```python
from build123d import *

# Parameters (mm, degrees)
SKETCH_1_R          = 17.75
EXTRUDE_1_DEPTH     = 1.6
SKETCH_2_R          = 2
EXTRUDE_2_DEPTH     = 11.3
EXTRUDE_START       = 1.6
SKETCH_3_R          = 17.75
EXTRUDE_3_DEPTH     = 1.6
CUT_EXTRUDE_2_REACH = 30.989
SKETCH_5_R          = 3.5
SKETCH_5_R_2        = 1
SKETCH_6_R          = 6
EXTRUDE_4_DEPTH     = 10
SKETCH_7_R          = 3
EXTRUDE_5_DEPTH     = 15
CHAMFER_1_SIZE      = 0.5
CUT_EXTRUDE_START   = -12
CUT_EXTRUDE_3_DEPTH = 12
SKETCH_10_R         = 3
EXTRUDE_6_DEPTH     = 2.8
EXTRUDE_7_REACH     = 39.456
SKETCH_13_R         = 1.9
CUT_EXTRUDE_4_REACH = 48.801
CUT_EXTRUDE_5_REACH = 48.801
SKETCH_17_R         = 1.25
CHAMFER_2_SIZE      = 0.5
EXTRUDE_START_2     = 1.2
SKETCH_19_R         = 3
EXTRUDE_8_DEPTH     = 1.2
EXTRUDE_9_REACH     = 39.456
SKETCH_20_R         = 1.9
SKETCH_21_R         = 3
EXTRUDE_10_DEPTH    = 1.2
CUT_EXTRUDE_START_2 = -10
SKETCH_22_R         = 6
SKETCH_22_R_2       = 3
CUT_EXTRUDE_6_DEPTH = 10
SKETCH_24_R         = 3
CUT_EXTRUDE_8_DEPTH = 12


with BuildPart() as part:
    # ｽｹｯﾁ1 → ﾎﾞｽ - 押し出し1 (new body)
    with BuildSketch(Plane.XY):
        Circle(SKETCH_1_R)
    extrude(amount=EXTRUDE_1_DEPTH)

    # ｽｹｯﾁ2 → ﾎﾞｽ - 押し出し2 (add)
    with BuildSketch(Plane(origin=(0, 0, 0), x_dir=(-1, 0, 0), z_dir=(0, 0, -1))):
        with Locations(Location((0, -15.5, 0), (0, 0, 180))):
            Circle(SKETCH_2_R)
        with Locations(Location((-13.423393759, 7.75, 0), (0, 0, 180))):
            Circle(SKETCH_2_R)
        with Locations(Location((13.423393759, 7.75, 0), (0, 0, 180))):
            Circle(SKETCH_2_R)
    extrude(amount=EXTRUDE_2_DEPTH)

    # ｽｹｯﾁ3 → ﾎﾞｽ - 押し出し3 (add)
    with BuildSketch(Plane(origin=(0, 0, -11.3), x_dir=(-1, 0, 0), z_dir=(0, 0, -1)).offset(EXTRUDE_START)):
        with Locations(Location((0, 0, 0), (0, 0, 180))):
            Circle(SKETCH_3_R)
    extrude(amount=-EXTRUDE_3_DEPTH)

    # ｽｹｯﾁ5 → ｶｯﾄ - 押し出し2 (cut, up to next)
    with BuildSketch(Plane(origin=(0, 0, -12.9), x_dir=(-1, 0, 0), z_dir=(0, 0, -1)), mode=Mode.PRIVATE) as cut_extrude_2_sk1:
        Circle(SKETCH_5_R)
    cut_extrude_2_tool1 = extrude(cut_extrude_2_sk1.sketch, amount=-CUT_EXTRUDE_2_REACH, mode=Mode.PRIVATE) & part.part
    # ｽｹｯﾁ5 → ｶｯﾄ - 押し出し2 (cut, up to next)
    with BuildSketch(Plane(origin=(0, 0, -12.9), x_dir=(-1, 0, 0), z_dir=(0, 0, -1)), mode=Mode.PRIVATE) as cut_extrude_2_sk2:
        with Locations((-13.423393759, 7.75)):
            Circle(SKETCH_5_R_2)
    cut_extrude_2_tool2 = extrude(cut_extrude_2_sk2.sketch, amount=-CUT_EXTRUDE_2_REACH, mode=Mode.PRIVATE) & part.part
    # ｽｹｯﾁ5 → ｶｯﾄ - 押し出し2 (cut, up to next)
    with BuildSketch(Plane(origin=(0, 0, -12.9), x_dir=(-1, 0, 0), z_dir=(0, 0, -1)), mode=Mode.PRIVATE) as cut_extrude_2_sk3:
        with Locations((13.423393759, 7.75)):
            Circle(SKETCH_5_R_2)
    cut_extrude_2_tool3 = extrude(cut_extrude_2_sk3.sketch, amount=-CUT_EXTRUDE_2_REACH, mode=Mode.PRIVATE) & part.part
    # ｽｹｯﾁ5 → ｶｯﾄ - 押し出し2 (cut, up to next)
    with BuildSketch(Plane(origin=(0, 0, -12.9), x_dir=(-1, 0, 0), z_dir=(0, 0, -1)), mode=Mode.PRIVATE) as cut_extrude_2_sk4:
        with Locations((0, -15.5)):
            Circle(SKETCH_5_R_2)
    cut_extrude_2_tool4 = extrude(cut_extrude_2_sk4.sketch, amount=-CUT_EXTRUDE_2_REACH, mode=Mode.PRIVATE) & part.part
    add(cut_extrude_2_tool1.solids().sort_by_distance((0, 0, -12.9))[0], mode=Mode.SUBTRACT)
    add(cut_extrude_2_tool2.solids().sort_by_distance((13.423394, 7.75, -12.9))[0], mode=Mode.SUBTRACT)
    add(cut_extrude_2_tool3.solids().sort_by_distance((-13.423394, 7.75, -12.9))[0], mode=Mode.SUBTRACT)
    add(cut_extrude_2_tool4.solids().sort_by_distance((0, -15.5, -12.9))[0], mode=Mode.SUBTRACT)

    # ｽｹｯﾁ6 → ﾎﾞｽ - 押し出し4 (add)
    with BuildSketch(Plane.XY.offset(1.6)):
        with Locations((0, 7)):
            Circle(SKETCH_6_R)
    extrude(amount=EXTRUDE_4_DEPTH)

    # ｽｹｯﾁ7 → ﾎﾞｽ - 押し出し5 (add)
    with BuildSketch(Plane.XY.offset(11.6)):
        with Locations((0, 7)):
            Circle(SKETCH_7_R)
    extrude(amount=EXTRUDE_5_DEPTH)

    # 面取り1
    chamfer_1_edges = [part.edges().sort_by_distance(p)[0] for p in [
        (-3, 7, 26.6),
    ]]
    chamfer(chamfer_1_edges, length=CHAMFER_1_SIZE)

    # ｽｹｯﾁ8 → ｶｯﾄ - 押し出し3 (cut)
    with BuildSketch(Plane.XY.offset(26.6).offset(CUT_EXTRUDE_START)):
        with BuildLine():
            Line((1.658312395, 9.5), (-1.658312395, 9.5))
            ThreePointArc((-1.658312395, 9.5), (0, 10), (1.658312395, 9.5))
        make_face()
    extrude(amount=CUT_EXTRUDE_3_DEPTH, mode=Mode.SUBTRACT)

    # ｽｹｯﾁ10 → ﾎﾞｽ - 押し出し6 (add)
    with BuildSketch(Plane.XY.offset(1.6)):
        with Locations((0, -5.5)):
            Circle(SKETCH_10_R)
        with Locations((9.5, -2.377501001)):
            Circle(SKETCH_10_R)
        with Locations((-9.5, -2.377501001)):
            Circle(SKETCH_10_R)
    extrude_6 = extrude(amount=-EXTRUDE_6_DEPTH)

    # ﾐﾗｰ1: ﾎﾞｽ - 押し出し6 across plane
    add(extrude_6.mirror(Plane.XY.offset(-5.65)))

    # ｽｹｯﾁ13 → ﾎﾞｽ - 押し出し7 (add, up to next)
    with BuildSketch(Plane(origin=(0, 0, -1.2), x_dir=(-1, 0, 0), z_dir=(0, 0, -1)), mode=Mode.PRIVATE) as extrude_7_sk1:
        with Locations(Location((-9.5, -2.377501001, 0), (0, 0, 180))):
            Circle(SKETCH_13_R)
    extrude_7_tool1 = extrude(extrude_7_sk1.sketch, amount=EXTRUDE_7_REACH, mode=Mode.PRIVATE) - part.part
    # ｽｹｯﾁ13 → ﾎﾞｽ - 押し出し7 (add, up to next)
    with BuildSketch(Plane(origin=(0, 0, -1.2), x_dir=(-1, 0, 0), z_dir=(0, 0, -1)), mode=Mode.PRIVATE) as extrude_7_sk2:
        with Locations(Location((0, -5.5, 0), (0, 0, 180))):
            Circle(SKETCH_13_R)
    extrude_7_tool2 = extrude(extrude_7_sk2.sketch, amount=EXTRUDE_7_REACH, mode=Mode.PRIVATE) - part.part
    # ｽｹｯﾁ13 → ﾎﾞｽ - 押し出し7 (add, up to next)
    with BuildSketch(Plane(origin=(0, 0, -1.2), x_dir=(-1, 0, 0), z_dir=(0, 0, -1)), mode=Mode.PRIVATE) as extrude_7_sk3:
        with Locations(Location((9.5, -2.377501001, 0), (0, 0, 180))):
            Circle(SKETCH_13_R)
    extrude_7_tool3 = extrude(extrude_7_sk3.sketch, amount=EXTRUDE_7_REACH, mode=Mode.PRIVATE) - part.part
    add(extrude_7_tool1.solids().sort_by_distance((9.5, -2.377501, -1.2))[0])
    add(extrude_7_tool2.solids().sort_by_distance((0, -5.5, -1.2))[0])
    add(extrude_7_tool3.solids().sort_by_distance((-9.5, -2.377501, -1.2))[0])

    # ｽｹｯﾁ15 → ｶｯﾄ - 押し出し4 (cut, up to next)
    with BuildSketch(Plane(origin=(0, 0, -12.9), x_dir=(-1, 0, 0), z_dir=(0, 0, -1)), mode=Mode.PRIVATE) as cut_extrude_4_sk1:
        with BuildLine():
            Line((2.236067977, -3.5), (-2.236067977, -3.5))
            ThreePointArc((-2.236067977, -3.5), (-1.99347124, -3.258109634), (-1.724878724, -3.045454545))
            ThreePointArc((-1.724878724, -3.045454545), (0, -2.5), (1.724878724, -3.045454545))
            ThreePointArc((1.724878724, -3.045454545), (1.99347124, -3.258109634), (2.236067977, -3.5))
        make_face()
    cut_extrude_4_tool1 = extrude(cut_extrude_4_sk1.sketch, amount=-CUT_EXTRUDE_4_REACH, mode=Mode.PRIVATE) & part.part
    add(cut_extrude_4_tool1.solids().sort_by_distance((0, -3.093671, -12.9))[0], mode=Mode.SUBTRACT)

    # ｽｹｯﾁ17 → ｶｯﾄ - 押し出し5 (cut, up to next)
    with BuildSketch(Plane(origin=(0, 0, -12.9), x_dir=(-1, 0, 0), z_dir=(0, 0, -1)), mode=Mode.PRIVATE) as cut_extrude_5_sk1:
        with Locations((-6.569553896, 13.48484192)):
            Circle(SKETCH_17_R)
    cut_extrude_5_tool1 = extrude(cut_extrude_5_sk1.sketch, amount=-CUT_EXTRUDE_5_REACH, mode=Mode.PRIVATE) & part.part
    # ｽｹｯﾁ17 → ｶｯﾄ - 押し出し5 (cut, up to next)
    with BuildSketch(Plane(origin=(0, 0, -12.9), x_dir=(-1, 0, 0), z_dir=(0, 0, -1)), mode=Mode.PRIVATE) as cut_extrude_5_sk2:
        with Locations((6.569553896, -13.48484192)):
            Circle(SKETCH_17_R)
    cut_extrude_5_tool2 = extrude(cut_extrude_5_sk2.sketch, amount=-CUT_EXTRUDE_5_REACH, mode=Mode.PRIVATE) & part.part
    add(cut_extrude_5_tool1.solids().sort_by_distance((6.569554, 13.484842, -12.9))[0], mode=Mode.SUBTRACT)
    add(cut_extrude_5_tool2.solids().sort_by_distance((-6.569554, -13.484842, -12.9))[0], mode=Mode.SUBTRACT)

    # 面取り2
    chamfer_2_edges = [part.edges().sort_by_distance(p)[0] for p in [
        (-6, 7, 11.6),
    ]]
    chamfer(chamfer_2_edges, length=CHAMFER_2_SIZE)

    # ｽｹｯﾁ19 → ﾎﾞｽ - 押し出し8 (add)
    with BuildSketch(Plane(origin=(0, 0, 0), x_dir=(-1, 0, 0), z_dir=(0, 0, -1)).offset(EXTRUDE_START_2)):
        with Locations(Location((0, 7, 0), (0, 0, 56.442690238))):
            Circle(SKETCH_19_R)
    extrude(amount=-EXTRUDE_8_DEPTH)

    # ｽｹｯﾁ20 → ﾎﾞｽ - 押し出し9 (add, up to next)
    with BuildSketch(Plane(origin=(0, 0, -1.2), x_dir=(-1, 0, 0), z_dir=(0, 0, -1)), mode=Mode.PRIVATE) as extrude_9_sk1:
        with Locations(Location((0, 7, 0), (0, 0, 180))):
            Circle(SKETCH_20_R)
    extrude_9_tool1 = extrude(extrude_9_sk1.sketch, amount=EXTRUDE_9_REACH, mode=Mode.PRIVATE) - part.part
    add(extrude_9_tool1.solids().sort_by_distance((0, 7, -1.2))[0])

    # ｽｹｯﾁ21 → ﾎﾞｽ - 押し出し10 (add)
    with BuildSketch(Plane.XY.offset(-11.3)):
        with Locations(Location((0, 7, 0), (0, 0, 123.557309762))):
            Circle(SKETCH_21_R)
    extrude(amount=EXTRUDE_10_DEPTH)

    # ｽｹｯﾁ22 → ｶｯﾄ - 押し出し6 (cut)
    with BuildSketch(Plane.XY.offset(11.6).offset(CUT_EXTRUDE_START_2)):
        with Locations((0, 7)):
            Circle(SKETCH_22_R)
        with Locations((0, 7)):
            Circle(SKETCH_22_R_2, mode=Mode.SUBTRACT)
    extrude(amount=CUT_EXTRUDE_6_DEPTH, mode=Mode.SUBTRACT)

    # ｽｹｯﾁ24 → ｶｯﾄ - 押し出し8 (cut)
    with BuildSketch(Plane.XY.offset(26.6).offset(CUT_EXTRUDE_START)):
        with Locations((0, 7)):
            Circle(SKETCH_24_R)
    extrude(amount=CUT_EXTRUDE_8_DEPTH, mode=Mode.SUBTRACT)


solid = part.part
```
Geometry check sheet. Reference: the model listing, model coordinates, mm. A direction names the side the tool comes from. Coordinates: 2 decimals unless noted, no trailing zeros. Order: outer loops, then holes, each group sorted by start corner. A loop starts at its lowest first (then second) coordinate and runs counter-clockwise, first axis right, second up. Notation, with made-up numbers: (-36.75, 79) - (-7.75, 79) arc R9 ccw to (-7.75, 93) - close; hole circle Ø4 at (70, 80.5). An arc over 180 degrees is marked (long way). Answer as a JSON object with one key per item and string values. Group by question number.
Item 1: Sectioned sample at A-A, the plane z = -7.5. Give the number of separate pieces and of enclosed holes in the cut face, and give its area (3 significant figures).
Item 2: Scan lines: probe 1 along Z at (x, y) = (-13.5, -2.5); probe 2 along Z at (x, y) = (2.5, -5.5); probe 3 along X at (y, z) = (-4, -8.75). Record each from-to range of solid material in increasing order.
Item 3: Depth check by flat-ended pin: pin 1 Ø4 at (x, y) = (-4.5, 13) entering from +Z; pin 2 Ø5 at (y, z) = (-9.5, -4) entering from -X; pin 3 Ø5 at (y, z) = (4.5, 5.5) entering from +X. Enter the tip coordinate at first touch or a pass-through.
Item 4: Sectioned sample at C-C, the plane y = 0. Record the cut outline in (x, z).
Item 5: Sectioned sample at B-B, the plane y = -15.5. Record the cut outline in (x, z).
Item 6: Tool access check on faces 1 (the face through (-3, 7, 8)), 2 (the face through (12.27, -3.53, -10.71)). Record the directions out of +Z, -Z, +X, -X, +Y, -Y that give a thin tool (end or side, any length) a straight path to the whole face; none if there is none.
Item 7: Sectioned sample at D-D, the plane x = -9.5. Record the cut outline in (y, z).
Item 8: Draft check along Z on faces 3 (the face through (-0.2, 3.7, -11.3)), 4 (the face through (-0.1, 3.5, -12.1)), 5 (the face through (0, 4, -12.9)). Enter one of: +Z half, -Z half, draft (parallel to the pull), parting line (faces both ways), or undercut.
Resolved:
{
 "1": {"separate pieces": "7", "enclosed holes": "3", "area": "73.6 mm^2"},
 "2": {"probe 1": "-12.9 to -11.3, 0 to 1.6", "probe 2": "-12.9 to -10.1, -1.2 to 1.6", "probe 3": "-10.49 to -8.51, -1.17 to 1.17, 8.51 to 10.49"},
 "3": {"pin 1": "z = 1.6", "pin 2": "x = -1.17", "pin 3": "x = 3"},
 "4": {"outline": "(-17.75, -12.9) - (-3.5, -12.9) - (-3.5, -11.3) - (-7.67, -11.3) - (-7.67, -10.1) - (-11.33, -10.1) - (-11.33, -11.3) - (-17.75, -11.3) - close; (-17.75, 0) - (-11.33, 0) - (-11.33, -1.2) - (-7.67, -1.2) - (-7.67, 0) - (7.67, 0) - (7.67, -1.2) - (11.33, -1.2) - (11.33, 0) - (17.75, 0) - (17.75, 1.6) - (-17.75, 1.6) - close; (3.5, -12.9) - (17.75, -12.9) - (17.75, -11.3) - (11.33, -11.3) - (11.33, -10.1) - (7.67, -10.1) - (7.67, -11.3) - (3.5, -11.3) - close"},
 "5": {"outline": "(-8.65, -12.9) - (-1, -12.9) - (-1, 1.6) - (-8.65, 1.6) - (-8.65, 0) - (-2, 0) - (-2, -11.3) - (-8.65, -11.3) - close; (1, -12.9) - (8.65, -12.9) - (8.65, -11.3) - (2, -11.3) - (2, 0) - (8.65, 0) - (8.65, 1.6) - (1, 1.6) - close"},
 "6": {"face 1": "+Z", "face 2": "none"},
 "7": {"outline": "(-14.99, -12.9) - (14.99, -12.9) - (14.99, -11.3) - (0.62, -11.3) - (0.62, -10.1) - (-0.48, -10.1) - (-0.48, -1.2) - (0.62, -1.2) - (0.62, 0) - (14.99, 0) - (14.99, 1.6) - (-14.99, 1.6) - (-14.99, 0) - (-5.38, 0) - (-5.38, -1.2) - (-4.28, -1.2) - (-4.28, -10.1) - (-5.38, -10.1) - (-5.38, -11.3) - (-14.99, -11.3) - close"},
 "8": {"face 3": "undercut", "face 4": "draft", "face 5": "-Z half"}
}
